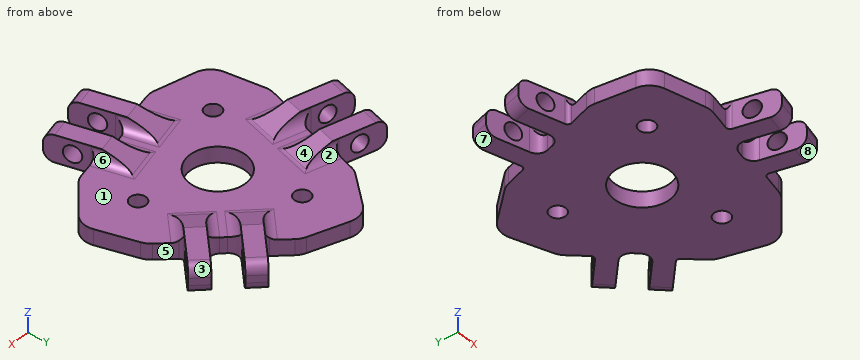
from build123d import *

# Parameters (mm, degrees)
SKETCH1_R                = 1.6
SKETCH1_R_2              = 5.6
BOSS_EXTRUDE1_DEPTH      = 3.175
SKETCH4_R                = 1.675
BOSS_EXTRUDE3_DEPTH      = 6.25
SKETCH4_2_R              = 1.675
CUT_EXTRUDE2_DEPTH       = 2.63125
FILLET1_R                = 2
FILLET2_R                = 2
FILLET3_R                = 2
CIRPATTERN2_COUNT        = 3
FILLET1_OF_CIRPATTERN2_R = 2
FILLET2_OF_CIRPATTERN2_R = 2
FILLET3_OF_CIRPATTERN2_R = 2
FILLET5_R                = 0.75


with BuildPart() as part:
    # Sketch1 → Boss-Extrude1 (new body)
    with BuildSketch(Plane.XY):
        with BuildLine():
            Line((15.347308801, 31.210973101), (8.051491314, 33.998880179))
            ThreePointArc((8.051491314, 33.998880179), (5.696175566, 34.15336703), (3.663829908, 32.952971436))
            Line((3.663829908, 32.952971436), (-1.653149933, 27.103867562))
            ThreePointArc((-1.653149933, 27.103867562), (-2.154824203, 26.417727613), (-2.500196213, 25.641078866))
            Line((-2.500196213, 25.641078866), (-9.325438013, 4.478720632))
            ThreePointArc((-9.325438013, 4.478720632), (-9.502063256, 3.613546149), (-9.484560317, 2.730700176))
            Line((-9.484560317, 2.730700176), (-8.507421128, -4.718687488))
            ThreePointArc((-8.507421128, -4.718687488), (-7.54564448, -6.839386894), (-5.565731281, -8.065080174))
            Line((-5.565731281, -8.065080174), (2.031002829, -10.077591551))
            ThreePointArc((2.031002829, -10.077591551), (2.960636861, -10.209852347), (3.895489669, -10.121746843))
            Line((3.895489669, -10.121746843), (25.485057009, -5.483666514))
            ThreePointArc((25.485057009, -5.483666514), (26.373611638, -5.180049941), (27.166902489, -4.677653705))
            Line((27.166902489, -4.677653705), (33.329625608, 0.328323939))
            ThreePointArc((33.329625608, 0.328323939), (34.614533997, 2.205289229), (34.668387555, 4.479291881))
            Line((34.668387555, 4.479291881), (32.591741985, 12.142614371))
            ThreePointArc((32.591741985, 12.142614371), (32.241466178, 13.013831458), (31.697738169, 13.779384986))
            Line((31.697738169, 13.779384986), (16.88625911, 30.157458595))
            ThreePointArc((16.88625911, 30.157458595), (16.17904213, 30.77516119), (15.347308801, 31.210973101))
        make_face()
        with Locations((24.879793107, 5.344918551)):
            Circle(SKETCH1_R, mode=Mode.SUBTRACT)
        with Locations((7.811061307, 24.218992148)):
            Circle(SKETCH1_R, mode=Mode.SUBTRACT)
        Circle(SKETCH1_R, mode=Mode.SUBTRACT)
        with Locations((10.896951472, 9.8546369)):
            Circle(SKETCH1_R_2, mode=Mode.SUBTRACT)
    extrude(amount=BOSS_EXTRUDE1_DEPTH)

    # Sketch4 → Boss-Extrude3 (add, symmetric)
    with BuildSketch(Plane(origin=(0.449621982, -0.475334512, 0), x_dir=(-0.726482741, -0.687184711, 0), z_dir=(0.687184711, -0.726482741, 0))):
        Polygon((-31.72132028, 0), (-31.72132028, -3.175), (-25.539496086, -3.175), (-31.72132028, -5.425), (-41.88132028, -5.425), (-41.88132028, 0), align=None)
        with Locations((-36.80132028, -2.7125)):
            Circle(SKETCH4_R, mode=Mode.SUBTRACT)
    boss_extrude3 = extrude(amount=BOSS_EXTRUDE3_DEPTH, both=True)

    # Sketch4<2> → Cut-Extrude2 (cut, symmetric)
    with BuildSketch(Plane(origin=(0.449621982, -0.475334512, 0), x_dir=(-0.726482741, -0.687184711, 0), z_dir=(0.687184711, -0.726482741, 0))):
        Polygon((-31.72132028, 0), (-31.72132028, -3.175), (-25.539496086, -3.175), (-31.72132028, -5.425), (-41.88132028, -5.425), (-41.88132028, 0), align=None)
        with Locations((-36.80132028, -2.7125)):
            Circle(SKETCH4_2_R, mode=Mode.SUBTRACT)
    cut_extrude2 = extrude(amount=CUT_EXTRUDE2_DEPTH, both=True, mode=Mode.SUBTRACT)

    # Fillet1
    fillet1_edges = [part.edges().sort_by_distance(p)[0] for p in [
        (19.440964609, 21.110601986, 3.175),
        (23.057274153, 17.287486564, 3.175),
        (25.865326768, 14.96244967, 3.175),
        (17.377217607, 24.139682361, 3.175),
        (22.0551547, 13.848979318, 3.175),
        (15.952095481, 20.301054157, 3.175),
    ]]
    fillet(fillet1_edges, radius=FILLET1_R)

    # Fillet2
    fillet2_edges = [part.edges().sort_by_distance(p)[0] for p in [
        (25.302768444, 19.411514101, 1.5875),
        (21.6864589, 23.234629523, 1.5875),
    ]]
    fillet(fillet2_edges, radius=FILLET2_R)

    # Fillet3
    fillet3_edges = [part.edges().sort_by_distance(p)[0] for p in [
        (33.927207925, 25.078831062, 0),
        (33.927207925, 25.078831062, 5.425),
        (27.824148706, 31.530905901, 5.425),
        (27.824148706, 31.530905901, 0),
    ]]
    fillet(fillet3_edges, radius=FILLET3_R)

    # CirPattern2: Boss-Extrude3, Cut-Extrude2 ×3 about axis
    cirpattern2_axis = Axis((10.896951472, 9.8546369, 0), (0, 0, 1))
    for i in range(1, CIRPATTERN2_COUNT):
        add(boss_extrude3.rotate(cirpattern2_axis, i * 360 / CIRPATTERN2_COUNT))
        add(cut_extrude2.rotate(cirpattern2_axis, i * 360 / CIRPATTERN2_COUNT), mode=Mode.SUBTRACT)

    # Fillet1 of CirPattern2
    fillet1_of_cirpattern2_edges = [part.edges().sort_by_distance(p)[0] for p in [
        (-3.123006806, 11.625986784, 3.175),
        (-1.620246501, 16.669360428, 3.175),
        (-1.010731793, 20.263723774, 3.175),
        (-4.71439386, 8.324189266, 3.175),
        (1.858647852, 17.520753147, 3.175),
        (-0.677483256, 9.009311403, 3.175),
        (16.372896612, -3.172678071, 3.175),
        (11.253826762, -4.392936293, 3.175),
        (7.836259441, -5.662262745, 3.175),
        (20.028030667, -2.899960928, 3.175),
        (8.777051863, -1.805821766, 3.175),
        (17.41624219, 0.253545139, 3.175),
    ]]
    fillet(fillet1_of_cirpattern2_edges, radius=FILLET1_OF_CIRPATTERN2_R)

    # Fillet2 of CirPattern2
    fillet2_of_cirpattern2_edges = [part.edges().sort_by_distance(p)[0] for p in [
        (-4.582455452, 17.552001759, 1.5875),
        (-6.085215757, 12.508628115, 1.5875),
        (11.970541423, -7.399605162, 1.5875),
        (17.089611272, -6.17934694, 1.5875),
    ]]
    fillet(fillet2_of_cirpattern2_edges, radius=FILLET2_OF_CIRPATTERN2_R)

    # Fillet3 of CirPattern2
    fillet3_of_cirpattern2_edges = [part.edges().sort_by_distance(p)[0] for p in [
        (-13.802715652, 22.187326963, 0),
        (-13.802715652, 22.187326963, 5.425),
        (-16.33884676, 13.675885219, 5.425),
        (-16.33884676, 13.675885219, 0),
        (12.566362141, -17.702247326, 0),
        (12.566362141, -17.702247326, 5.425),
        (21.205552469, -15.642880421, 5.425),
        (21.205552469, -15.642880421, 0),
    ]]
    fillet(fillet3_of_cirpattern2_edges, radius=FILLET3_OF_CIRPATTERN2_R)

    # Fillet5
    fillet5_edges = [part.edges().sort_by_distance(p)[0] for p in [
        (-7.789671487, 9.240521362, 1.5875),
        (-3.951849266, 21.140080535, 1.5875),
        (20.879758905, -6.473021336, 1.5875),
        (8.655527257, -9.099149384, 1.5875),
        (20.045714571, 26.663830856, 2.5875),
        (28.432123998, 17.390399731, 2.5875),
    ]]
    fillet(fillet5_edges, radius=FILLET5_R)


solid = part.part
For this review, take the finished solid that the model builds, in its own axes (mm). Face numbers are marked on the shaded views. A direction names the side the tool comes from. Coordinates: 2 decimals unless noted, no trailing zeros. Use a Markdown table: item, result. Add a question column.
Item 1: For line 1 (Y direction, x = 25.5, z = 3); line 2 (Y direction, x = 11, z = 2.15); line 3 (Z direction, x = 16, y = 7) (3 decimals), list the stretches that pass through material, from the lowest coordinate up.
Item 2: Tool access review of the marked faces 1, 2, 3, 4 and 5: name each direction out of +Z, -Z, +X, -X, +Y, -Y from which nothing blocks a thin tool from reaching the whole face with its end or side.
Item 3: Insertion check: pin 1 Ø1.5 at (x, z) = (12, 1) entering from +Y; pin 2 Ø3 at (y, z) = (6.5, 3) entering from +X; pin 3 Ø2 at (x, z) = (-1.5, 1.5) entering from -Y. Each pin has a flat end and moves straight along its axis. Give the tip position at first contact, or say it passes through.
Item 4: Mouldability with a two-part tool opening along Y and no side actions: class the marked faces 6, 7 and 8 as pulls with the +Y half, pulls with the -Y half, needs draft (parallel to the pull), parting line crosses it, or undercut.
Results list:
| question | item | result |
|---|---|---|
| 1 | line 1 | y = -5.48 to 3.87, 6.82 to 20.24, 29 to 31.82 |
| 1 | line 2 | y = -18.08 to -14.48, -11.23 to 4.26, 15.45 to 32.87 |
| 1 | line 3 | z = 0 to 3.175 |
| 2 | face 1 | +Z |
| 2 | face 2 | +Z, +Y |
| 2 | face 3 | +Z, +X, +Y |
| 2 | face 4 | +Z, -Y |
| 2 | face 5 | +Z, -Z, +X |
| 3 | pin 1 | stops at y = 32.78 |
| 3 | pin 2 | stops at x = 34.53 |
| 3 | pin 3 | stops at y = -9.41 |
| 4 | face 6 | undercut |
| 4 | face 7 | pulls with the +Y half |
| 4 | face 8 | pulls with the -Y half |
